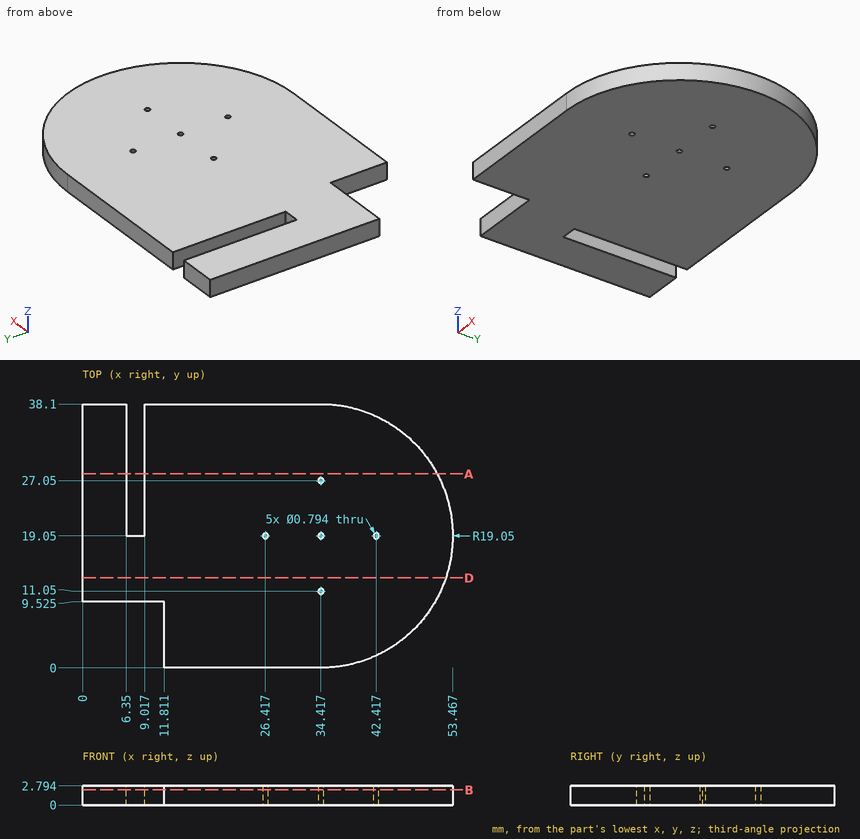
The figure shows three views and two pictorial views of one solid part (mm, origin at its lowest corner). Answer the questions. Round coordinates to 2 decimals unless told otherwise and drop trailing zeros. Order: outer loops, then holes, each group sorted by start corner. A loop starts at its lowest first (then second) coordinate and runs counter-clockwise, first axis right, second up. Notation, with made-up numbers: (51, -7.75) - (88, -7.75) arc R17 cw to (88, 24.25) - close; hole circle Ø2 at (-7.75, 31.5). An arc over 180 degrees is marked (long way). Write item = value, one per line. Start each with the question number.
1) Section A-A, the plane y = 28 is taken. Write down the section's boundary in (x, z).
2) Section D-D, the plane y = 13 is taken. Write down the section's boundary in (x, z).
3) Straight lines are drawn through the part: L1, parallel to X at y = 28, z = 2.4; L2, parallel to X at y = 31, z = 0.7; L3, parallel to X at y = 5, z = 0.3. For each, find the intervals that lie inside material, in ascending order.
4) Section B-B, the plane z = 2.2 is taken. Count the separate pieces of the cut face and the enclosed holes in it, plus the area to 3 significant figures.
5) Given pin 1 (4 mm diameter, centred on x = 44, y = 21, fed in from -Z); pin 2 (1.4 mm diameter, centred on x = 4, z = 1.5, fed in from -Y) (3 decimals), each flat-ended and moving along its own axis, determine where each tip first touches the part or whether it passes through.
Results list:
q1.outline = (0, 0) - (6.35, 0) - (6.35, 2.79) - (0, 2.79) - close; (9.02, 0) - (51.23, 0) - (51.23, 2.79) - (9.02, 2.79) - close
q2.outline = (0, 0) - (52.48, 0) - (52.48, 2.79) - (0, 2.79) - close
q3.L1 = 0 to 6.35, 9.02 to 51.23
q3.L2 = 0 to 6.35, 9.02 to 49.25
q3.L3 = 11.81 to 47.28
q4.separate_pieces = 1
q4.enclosed_holes = 5
q4.area = 1,720 mm^2
q5.pin_1 = 0
q5.pin_2 = 9.525
